Autodesk Fusion 360 part; units mm, degrees
sketch "草图1" plane through (0, 0, 0) normal (0, 1, 0) x (1, 0, 0)
  line L0 (0, 0) -> (40.2, 0)
  line L1 (40.2, 0) -> (40.2, -20.2)
  line L2 (40.2, -20.2) -> (0, -20.2)
  line L3 (0, -20.2) -> (0, 0)
  dimension "d1" = 20.2
  dimension "d2" = 40.2
extrude "拉伸1" add sketch "草图1" along normal blind 40.1 makes body 1
sketch "草图2" plane through (0, 0, 0) normal (0, -1, 0) x (1, 0, 0)
  line L0 (40.2, 20.2) -> (0, 20.2)
  line L1 (0, 20.2) -> (0, 0)
  line L2 (0, 0) -> (40.2, 0)
  line L3 (40.2, 0) -> (40.2, 20.2)
  line L4 (20.1, 23) -> (20.1, -21)
  line L5 (2.071, 10.1) -> (35, 10.1)
  circle A0 centre (2.6, 17.6) radius 0.8
  circle A1 centre (37.6, 17.6) radius 0.8
  circle A2 centre (2.6, 2.6) radius 0.8
  circle A3 centre (37.6, 2.6) radius 0.8
  circle A4 centre (17.6, 17.6) radius 0.8
  circle A5 centre (17.6, 2.6) radius 0.8
  dimension "d5" = 1.6
  dimension "d6" = 15
  dimension "d7" = 35
  dimension "d8" = 1.6
  dimension "d9" = 5
  dimension "d12" = 15
extrude "拉伸2" cut sketch "草图2" against normal blind 4 contours A0 | A1 | A2 | A3 | A4 | A5 bodies 1
sketch "草图3" plane through (0, 0, 0) normal (0, -1, 0) x (1, 0, 0)
  circle A0 centre (17.6, 2.6) radius 0.8
  circle A1 centre (2.6, 17.6) radius 0.8
  circle A2 centre (37.6, 17.6) radius 0.8
  circle A3 centre (17.6, 17.6) radius 0.8
  circle A4 centre (2.6, 2.6) radius 0.8
  circle A5 centre (37.6, 2.6) radius 0.8
  line L0 (40.2, 20.2) -> (0, 20.2)
  line L1 (0, 20.2) -> (0, 0)
  line L2 (0, 0) -> (40.2, 0)
  line L3 (40.2, 0) -> (40.2, 20.2)
  line L4 (20.1, 18.9238) -> (20.1, 1)
  circle A6 centre (30.1, 9.9619) radius 6
  dimension "d13" = 12
  dimension "d29" = 20
extrude "拉伸3" add sketch "草图3" along normal blind 1.65 contours A6 bodies 1
sketch "草图4" plane through (0, -1.65, 0) normal (0, -1, 0) x (1, 0, 0)
  circle A0 centre (30.1, 9.9619) radius 6
  circle A1 centre (30.1, 9.9619) radius 3
  dimension "d16" = 6
extrude "拉伸4" add sketch "草图4" along normal blind 3.9 contours A1 bodies 1
sketch "草图5" plane through (0, 40.1, 0) normal (0, 1, 0) x (-1, 0, 0)
  line L0 (0, 20.2) -> (-40.2, 20.2)
  line L1 (-40.2, 20.2) -> (-40.2, 0)
  line L2 (-40.2, 0) -> (0, 0)
  line L3 (0, 0) -> (0, 20.2)
  line L4 (-20.1, 1) -> (-20.1, 25)
  circle A0 centre (-30.1, 10) radius 6
  dimension "d19" = 12
  dimension "d20" = 20
extrude "拉伸5" add sketch "草图5" along normal blind 1.65 contours A0 bodies 1
sketch "草图6" plane through (0, 41.75, 0) normal (0, 1, 0) x (-1, 0, 0)
  circle A0 centre (-30.1, 10) radius 6
  circle A1 centre (-30.1, 10) radius 3
  dimension "d23" = 6
extrude "拉伸6" add sketch "草图6" along normal blind 4.1 contours A1 bodies 1
sketch "草图7" plane through (0, 45.85, 0) normal (0, 1, 0) x (-1, 0, 0)
  circle A0 centre (-30.1, 10) radius 3
  circle A1 centre (-30.1, 10) radius 1.5
  dimension "d26" = 3
extrude "拉伸7" cut sketch "草图7" against normal blind 6 contours A1 bodies 1
sketch "草图8" plane through (0, 40.1, 0) normal (0, 1, 0) x (-1, 0, 0)
  circle A0 centre (-30.1, 10) radius 6
  line L0 (0, 20.2) -> (-40.2, 20.2)
  line L1 (-40.2, 20.2) -> (-40.2, 0)
  line L2 (-40.2, 0) -> (0, 0)
  line L3 (0, 0) -> (0, 20.2)
  line L4 (-20.1, 25.0001) -> (-20.1, -10.3333)
  circle A1 centre (-2.95, 10) radius 0.8
  line L5 (-39, 10) -> (5, 10)
  circle A2 centre (-9.95, 15.167) radius 0.8
  circle A3 centre (-9.95, 4.833) radius 0.8
  dimension "d30" = 1.6
  dimension "d31" = 34.3
  dimension "d32" = 1.6
  dimension "d33" = 7
extrude "拉伸8" cut sketch "草图8" against normal blind 6 contours A1 L5 | A1 L5 | A2 | A3 bodies 1
fillet "圆角1" radius 1 12 edges at (40.2, 20.05, 20.2) (40.2, 40.1, 10.1) (40.2, 20.05, 0) (40.2, 0, 10.1) (20.1, 40.1, 0) (20.1, 40.1, 20.2) (20.1, 0, 20.2) (20.1, 0, 0) (0, 20.05, 20.2) (0, 40.1, 10.1) (0, 20.05, 0) (0, 0, 10.1) on bodies 1
sketch "草图9" plane through (0, -5.55, 0) normal (0, -1, 0) x (1, 0, 0)
  circle A0 centre (30.1, 9.9619) radius 3
  circle A1 centre (30.1, 9.9619) radius 1.5
  dimension "d38" = 3
extrude "拉伸9" cut sketch "草图9" against normal blind 6 contours A1 bodies 1
copy_body "实体->零部件1" bodies 1 removing the originals makes body 2 in component "Component'"
component "Component'" placed x (1, 0, 0) y (0, 1, 0) z (0, 0, 1) at (0, 0, 0)
Source: CAD feature listing. Evaluate the final solid. Frame: model axes, mm. A direction names the side the tool comes from. Give positions to 0.01 mm unless a question says otherwise; leave off trailing zeros. Order: outer loops, then holes, each group sorted by start corner. A loop starts at its lowest first (then second) coordinate and runs counter-clockwise, first axis right, second up. Notation, with made-up numbers: (45, 52.5) -> (88, 52.5) arc R24 ccw to (88, 82.5) -> close; hole circle Ø1 at (-4.75, -22.5). An arc over 180 degrees is marked (long way). Use a Markdown table: item, result.
Q1. Section A-A (x = 17.6). Return the cut outline in (y, z).
A:
| item | result |
|---|---|
| outline | (0, 1) arc R1 ccw to (1, 0) -> (39.1, 0) arc R1 ccw to (40.1, 1) -> (40.1, 19.2) arc R1 ccw to (39.1, 20.2) -> (1, 20.2) arc R1 ccw to (0, 19.2) -> (0, 18.4) -> (4, 18.4) -> (4, 16.8) -> (0, 16.8) -> (0, 3.4) -> (4, 3.4) -> (4, 1.8) -> (0, 1.8) -> close |
Q2. First-contact query: P1, Ø1.5, axis at x = 26.5, z = 13, coming from the -Y side; P2, Ø4, axis at x = 22.5, z = 5.5, coming from the +Y side; P3, Ø3, axis at y = 8, z = 3, coming from the -X side; P4, Ø1, axis at x = 2.95, z = 10, coming from the +Y side. Flat tips, straight axial feed; report the tip coordinate or a pass-through.
A:
| item | result |
|---|---|
| P1 | y = -1.65 |
| P2 | y = 40.1 |
| P3 | x = 0 |
| P4 | y = 34.1 |
Q3. Pull-direction query (Z, two-part tool) for faces 4 (the face through (20, 20, 0)), 5 (the face through (38, 4, 3)), 6 (the face through (33.326, -0.813, 4.903)); classes: +Z half, -Z half, draft (parallel to the pull), parting line (faces both ways), or undercut.
A:
| item | result |
|---|---|
| face 4 | -Z half |
| face 5 | undercut |
| face 6 | parting line |
Q4. Material intervals for line 1 (Z direction, x = 17, y = 1); line 2 (Y direction, x = 22, z = 2.75); line 3 (Z direction, x = 30.1, y = -4), sorted ascending. Write a range as [from, to].
A:
| item | result |
|---|---|
| line 1 | [0, 2.07], [3.13, 17.07], [18.13, 20.2] |
| line 2 | [0, 40.1] |
| line 3 | [6.96, 8.46], [11.46, 12.96] |
Q5. Section B-B (x = 32.5). Return the cut outline in (y, z).
A:
| item | result |
|---|---|
| outline | (-5.55, 8.16) -> (-1.65, 8.16) -> (-1.65, 4.46) -> (0, 4.46) -> (0, 1) arc R1 ccw to (1, 0) -> (39.1, 0) arc R1 ccw to (40.1, 1) -> (40.1, 4.5) -> (41.75, 4.5) -> (41.75, 8.2) -> (45.85, 8.2) -> (45.85, 11.8) -> (41.75, 11.8) -> (41.75, 15.5) -> (40.1, 15.5) -> (40.1, 19.2) arc R1 ccw to (39.1, 20.2) -> (1, 20.2) arc R1 ccw to (0, 19.2) -> (0, 15.46) -> (-1.65, 15.46) -> (-1.65, 11.76) -> (-5.55, 11.76) -> close |
Q6. Access query for faces 1 (the face through (28.8, 45.85, 8.7)), 2 (the face through (30, 39.85, 10)), 3 (the face through (18, 4, 18)). Directions: +Z, -Z, +X, -X, +Y, -Y. A direction counts if a zero-diameter tool reaches every point of the face in a straight line with its end or side. Return the directions, or none.
A:
| item | result |
|---|---|
| face 1 | +Z, -Z, +X, -X, +Y |
| face 2 | +Y |
| face 3 | -Y |
